Design review of the part built by this model. Coordinates are the model's own, in mm. A direction names the side the tool comes from. Coordinates: 2 decimals unless noted, no trailing zeros. Write each loop counter-clockwise with the first axis right and the second up, starting at its lowest first coordinate (ties: lowest second). Pieces come first, ordered by that corner, then holes.
```python
from build123d import *

# Parameters (mm, degrees)
BOSS_EXTRUDE1_DEPTH = 2.5
BOSS_EXTRUDE2_DEPTH = 15


with BuildPart() as part:
    # Sketch1 → Boss-Extrude1 (new body)
    with BuildSketch(Plane(origin=(0, 0, 0), x_dir=(1, 0, 0), z_dir=(0, 1, 0))):
        Polygon((461.073568615, -149.83773521), (452.699844164, -164.341477869), (443.467960434, -148.412314407), (460.250524065, -148.418039508), align=None)
        Polygon((443.467960434, -148.412314407), (443.467960434, -135.912167949), (460.250524065, -135.906442848), (461.073568615, -134.486747146), (452.699844164, -119.983004487), (463.501448438, -113.746497393), (471.875594509, -128.249996622), (473.516609246, -128.247021872), (481.912449677, -113.71552717), (492.738048515, -119.96567817), (484.351348131, -134.502449871), (485.169281539, -135.925096404), (501.916753351, -135.925543562), (501.91660162, -148.398260812), (485.169129802, -148.398300503), (484.351161781, -149.820927135), (492.737508483, -164.357902881), (481.912073973, -170.607993214), (473.515811116, -156.076742585), (471.874796293, -156.07381554), (463.501071842, -170.577558199), (452.699844164, -164.341477869), (461.073568615, -149.83773521), (460.250524065, -148.418039508), align=None)
        Polygon((461.073568615, -134.486747146), (460.250524065, -135.906442848), (443.467960434, -135.912167949), (452.699844164, -119.983004487), align=None)
        Polygon((471.874796293, -156.07381554), (473.515811116, -156.076742585), (481.912073973, -170.607993214), (463.501071842, -170.577558199), align=None)
        Polygon((485.169129802, -148.398300503), (501.91660162, -148.398260812), (492.737508483, -164.357902881), (484.351161781, -149.820927135), align=None)
        Polygon((485.169281539, -135.925096404), (484.351348131, -134.502449871), (492.738048515, -119.96567817), (501.916753351, -135.925543562), align=None)
        Polygon((471.875594509, -128.249996622), (463.501448438, -113.746497393), (481.912449677, -113.71552717), (473.516609246, -128.247021872), align=None)
    extrude(amount=-BOSS_EXTRUDE1_DEPTH)

    # Sketch1_12 → Boss-Extrude2 (add)
    with BuildSketch(Plane(origin=(0, 0, 0), x_dir=(1, 0, 0), z_dir=(0, 1, 0))):
        Polygon((471.874796293, -156.07381554), (473.515811116, -156.076742585), (481.912073973, -170.607993214), (463.501071842, -170.577558199), align=None)
        Polygon((461.073568615, -149.83773521), (452.699844164, -164.341477869), (443.467960434, -148.412314407), (460.250524065, -148.418039508), align=None)
        Polygon((461.073568615, -134.486747146), (460.250524065, -135.906442848), (443.467960434, -135.912167949), (452.699844164, -119.983004487), align=None)
        Polygon((471.875594509, -128.249996622), (463.501448438, -113.746497393), (481.912449677, -113.71552717), (473.516609246, -128.247021872), align=None)
        Polygon((485.169281539, -135.925096404), (484.351348131, -134.502449871), (492.738048515, -119.96567817), (501.916753351, -135.925543562), align=None)
        Polygon((485.169129802, -148.398300503), (501.91660162, -148.398260812), (492.737508483, -164.357902881), (484.351161781, -149.820927135), align=None)
    extrude(amount=BOSS_EXTRUDE2_DEPTH)


solid = part.part
```
(1) Consider section A-A (y = 8.25). Give the boundary of the cut face in (x, z), plus the area to 3 significant figures.
(2) Consider section D-D (z = 159.5). Give the boundary of the cut face in (x, y) (1 decimal), plus the area to 3 significant figures.
(3) Consider section B-B (z = 118.5). Give the boundary of the cut face in (x, y), plus the area to 3 significant figures.
(4) Insertion check: pin 1 Ø3 at (y, z) = (5, 153.5) entering from -X; pin 2 Ø8 at (x, y) = (494, 13) entering from -Z; pin 3 Ø2 at (y, z) = (9, 153.5) entering from +X. Each pin has a flat end and moves straight along its axis. Give the tip position at first contact, or say it passes through.
(5) Wall thickness on line 1 (X direction, y = 6.5, z = 159); line 2 (X direction, y = 5.75, z = 122.5); line 3 (Y direction, x = 470, z = 155): over which ranges is each line inside the solid? List them lowest first.
(6) Mouldability with a two-part tool opening along X and no side actions: class faces 4 (the flat face through (443.468, -1, 142)), 5 (the flat face through (484.766, 7.395, 135.224)), 6 (the flat face through (493, 15, 130)) as +X half, -X half, draft (parallel to the pull), parting line (faces both ways), or undercut.
(7) For faces 1 (the flat face through (473, 0, 142)), 2 (the flat face through (456.828, 7.395, 127.133)), 3 (the flat face through (497.39, 6.37, 156.27)), list the 3-axis set-ups (+Z, -Z, +X, -X, +Y, -Y) from which the entire face can be reached by the end or side of a thin tool; tool diameter is ignored.
(8) Consider section C-C (x = 449.5). Give the boundary of the cut face in (y, z), plus the area to 3 significant figures.
Results:
1. outline: (443.47, 135.91) - (452.7, 119.98) - (461.07, 134.49) - (460.25, 135.91) - close; (443.47, 148.41) - (460.25, 148.42) - (461.07, 149.84) - (452.7, 164.34) - close; (463.5, 113.75) - (481.91, 113.72) - (473.52, 128.25) - (471.88, 128.25) - close; (463.5, 170.58) - (471.87, 156.07) - (473.52, 156.08) - (481.91, 170.61) - close; (484.35, 134.5) - (492.74, 119.97) - (501.92, 135.93) - (485.17, 135.93) - close; (484.35, 149.82) - (485.17, 148.4) - (501.92, 148.4) - (492.74, 164.36) - close
1. area: 873 mm2
2. outline: (449.9, -2.5) - (495.5, -2.5) - (495.5, 15) - (489.9, 15) - (489.9, 0) - (475.5, 0) - (475.5, 15) - (469.9, 15) - (469.9, 0) - (455.5, 0) - (455.5, 15) - (449.9, 15) - close
2. area: 366 mm2
3. outline: (455.27, -2.5) - (490.2, -2.5) - (490.2, 0) - (479.15, 0) - (479.15, 15) - (466.25, 15) - (466.25, 0) - (455.27, 0) - close
3. area: 281 mm2
4. pin 1: stops at x = 445.55
4. pin 2: stops at z = 119.97
4. pin 3: stops at x = 499.56
5. line 1: x = 449.6 to 455.78, 470.19 to 475.2, 489.65 to 495.82
5. line 2: x = 451.24 to 454.15, 468.56 to 476.84, 491.28 to 494.2
5. line 3: y = -2.5 to 0
6. face 4: -X half
6. face 5: undercut
6. face 6: draft
7. face 1: +Y
7. face 2: -Z, +Y
7. face 3: +Z, +X, +Y, -Y
8. outline: (-2.5, 125.5) - (15, 125.5) - (15, 135.91) - (0, 135.91) - (0, 148.41) - (15, 148.41) - (15, 158.82) - (-2.5, 158.82) - close
8. area: 395 mm2
